Can you work these out from the drawing? Everything is in mm from the part's minimum corner. Give positions to 0.01 mm unless a question says otherwise; leave off trailing zeros. Order: outer loops, then holes, each group sorted by start corner. A loop starts at its lowest first (then second) coordinate and runs counter-clockwise, first axis right, second up. Notation, with made-up numbers: M -2,20 L 11,20 A23 cw 11,45 Z; hole C 68.25,-12 d4. An arc over 180 degrees is marked long. Answer as a JSON object with one key per item and string values.
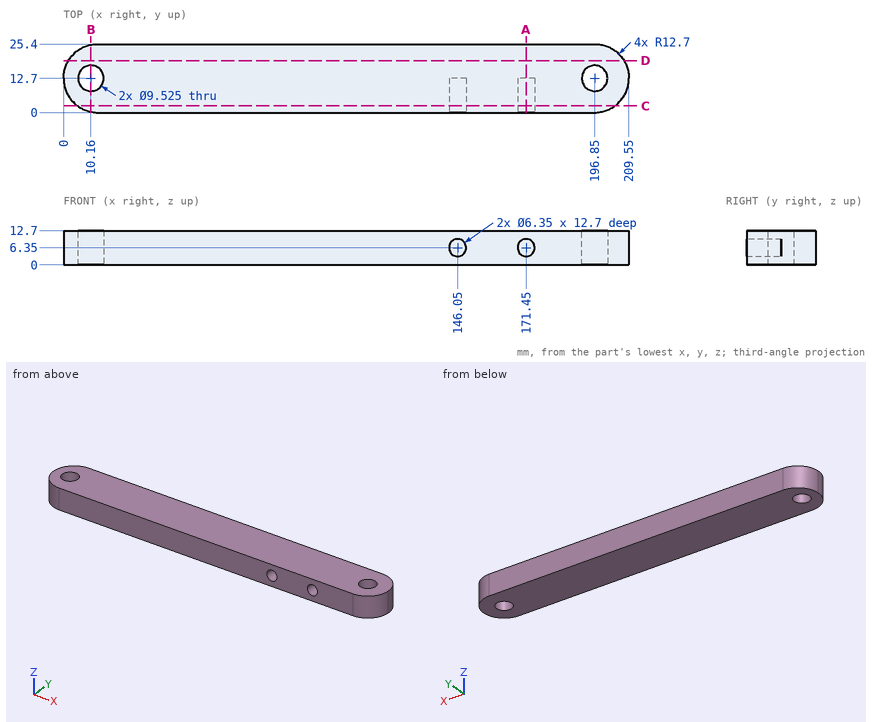
1) I want a section at C-C on y = 2.5. Count the separate pieces of the cut face and the enclosed holes in it, and give its area (3 significant figures).
Results found:
{"separate pieces": "1", "enclosed holes": "2", "area": "2,470 mm²"}
2) I want a section at D-D on y = 19.25. Write out the boundary of the cut face in (x, z), and give its area (4 significant figures).
Results found:
{"outline": "M 1.82,0 L 207.73,0 L 207.73,12.7 L 1.82,12.7 Z", "area": "2,615 mm²"}
3) I need wall thicknesses on L1, parallel to X at y = 12.5, z = 1.25; L2, parallel to X at y = 11.5, z = 6; L3, parallel to Z at x = 146.05, y = 7.75 (3 decimals). Which ranges of each line are inside material? Lowest first, please.
Results found:
{"L1": "x = 0 to 5.4, 14.92 to 192.09, 201.61 to 209.55", "L2": "x = 0.06 to 5.55, 14.77 to 142.89, 149.21 to 168.29, 174.61 to 192.24, 201.46 to 209.49", "L3": "z = 0 to 3.175, 9.525 to 12.7"}
4) I want a section at B-B on x = 10.16. Write out the boundary of the cut face in (y, z).
Results found:
{"outline": "M 0.26,0 L 7.94,0 L 7.94,12.7 L 0.26,12.7 Z; M 17.46,0 L 25.14,0 L 25.14,12.7 L 17.46,12.7 Z"}
5) I'm going to push flat-ended pins straight in: pin 1 Ø1.9 at (x, z) = (171, 5) entering from -Y; pin 2 Ø3 at (y, z) = (8.5, 6.5) entering from +X. Where does each tip first touch, or does it pass through?
Results found:
{"pin 1": "stops at y = 12.7", "pin 2": "stops at x = 209.26"}
6) I want a section at A-A on x = 171.45. Write out the boundary of the cut face in (y, z) (3 decimals).
Results found:
{"outline": "M 0,0 L 25.4,0 L 25.4,12.7 L 0,12.7 L 0,9.525 L 12.7,9.525 L 12.7,3.175 L 0,3.175 Z"}
